Part model, mm, in its own coordinate system. Face numbers are marked on the shaded views. A direction names the side the tool comes from. Round coordinates to 2 decimals unless told otherwise and drop trailing zeros. Write each loop counter-clockwise with the first axis right and the second up, starting at its lowest first coordinate (ties: lowest second). Pieces come first, ordered by that corner, then holes. Notation, with made-up numbers: (11, 84.5) -> (48, 84.5) arc R7 ccw to (48, 96.5) -> close; hole circle Ø2 at (-21, 26.5). An arc over 180 degrees is marked (long way). Return JSON: item names as keys, results as strings. Group by question number.
(1) Saw through at C-C (y = 0.3). List the corners of the cut face in (x, z).
(2) Drill centre lines: L1, parallel to Z at x = 0, y = 0.55; L2, parallel to X at y = 0.3, z = 4; L3, parallel to X at y = 0.95, z = -4. Where is each one in solid material? Low to high. Write a range as from..to.
(3) Saw through at D-D (x = 8). List the corners of the cut face in (y, z), plus the area to 3 significant figures.
(4) Tool access for the marked faces 1, 2, 3, 4 and 5: list every direction of +Z, -Z, +X, -X, +Y, -Y with a clear straight run to the whole face (end or side of a thin tool).
(5) Mould opens along Z. For the marked faces 6, 7 and 8 say: +Z half, -Z half, draft (parallel to the pull), parting line (faces both ways), or undercut.
(6) Saw through at B-B (z = -4). List the corners of the cut face in (x, y), plus the area to 3 significant figures.
(7) Saw through at A-A (z = 4). List the corners of the cut face in (x, y).
Autodesk Inventor part; units mm, degrees
ref_plane "YZ Plane" through (0, 0, 0) normal (1, 0, 0) x (0, 1, 0)
ref_plane "XZ Plane" through (0, 0, 0) normal (0, 1, 0) x (-1, 0, 0)
ref_plane "XY Plane" through (0, 0, 0) normal (0, 0, 1) x (1, 0, 0)
sketch "Sketch1" plane through (0, 0, 0) normal (0, 1, 0) x (-1, 0, 0)
  line L0 (-1.5, -4) -> (1.5, -4)
  line L1 (1.5, -4) -> (1.5, 4)
  line L2 (1.5, 4) -> (-1.5, 4)
  line L3 (-1.5, 2) -> (-1.5, -4)
  line L4 (-1.5, -4) -> (1.5, 4) construction
  line L5 (1.5, -4) -> (-1.5, 4) construction
  circle A0 centre (0, 4) radius 1.2
  circle A1 centre (0, -4) radius 1.2
  circle A2 centre (0, -4) radius 2
  circle A3 centre (0, 4) radius 2
  line L6 (-2, 2.5) -> (-8, 2.5)
  line L7 (-8, 2.5) -> (-8, 5.5)
  line L8 (-8, 5.5) -> (0, 5.5)
  line L9 (0, 5.5) -> (0, 2.5)
  circle A4 centre (-8, 4) radius 1.2
  circle A5 centre (-8, 4) radius 2
  arc A6 (-1.5, 2) -> (-2, 2.5) centre (-2, 2) ccw
  point P0 (0, 0)
  point P1 (-1.5, -2.6771)
  point P2 (1.5, -2.6771)
  point P3 (1.5, 2.6771)
  point P4 (-1.5, 2.6771)
  point P5 (-6.6771, 2.5)
  point P6 (-1.5, 2.5)
  point P7 (-1.3229, 5.5)
  point P8 (-6.6771, 5.5)
  point P9 (-8, 5.2)
  point P10 (-8, 2.8)
  dimension "d0" = 3
  dimension "linkPitchLength" = 8
  dimension "d3" = 2.4
  dimension "d4" = 4
  dimension "linkPitchWidth" = 8
  dimension "d17" = 0.5
extrude "Extrusion1" add sketch "Sketch1" along normal blind 1 contours A1 L0 L3 A2 L1 | L0 L1 A2 L3 A1 | A2 L3 A6 L6 A5 L8 A3 L1 | A3 L8 L9 A0 L2 L1 | L1 L2 A0 L9 L8 A3 | A5 L6 L7 A4 L8 | L8 L7 A4 L6 A5
sketch "Sketch2" plane through (0, 1, 0) normal (0, 1, 0) x (1, 0, 0)
  line L0 (6.6771, -2.5) -> (2, -2.5)
  arc A0 (1.5, -2) -> (2, -2.5) centre (2, -2) ccw
  line L1 (1.5, -2) -> (1.5, 2.6771)
  arc A1 (1.5, 2.6771) -> (-1.5, 2.6771) centre (0, 4) ccw
  line L2 (-1.5, 2.6771) -> (-1.5, -2.6771)
  arc A2 (-1.5, -2.6771) -> (1.3229, -5.5) centre (0, -4) ccw
  line L3 (1.3229, -5.5) -> (6.6771, -5.5)
  arc A3 (6.6771, -5.5) -> (6.6771, -2.5) centre (8, -4) ccw
  circle A4 centre (8, -4) radius 1.2
  circle A5 centre (0, 4) radius 1.2
  circle A6 centre (0, -4) radius 1.2
  point P0 (0, 0)
extrude "Extrusion2" [suppressed]
sketch "Sketch5" plane through (0, 1, 0) normal (0, 1, 0) x (1, 0, 0)
  line L0 (6.6771, -2.5) -> (2, -2.5)
  arc A0 (1.5, -2) -> (2, -2.5) centre (2, -2) ccw
  line L1 (1.5, -2) -> (1.5, 2.6771)
  arc A1 (1.5, 2.6771) -> (-1.5, 2.6771) centre (0, 4) ccw
  line L2 (-1.5, 2.6771) -> (-1.5, -2.6771)
  arc A2 (-1.5, -2.6771) -> (1.3229, -5.5) centre (0, -4) ccw
  line L3 (1.3229, -5.5) -> (6.6771, -5.5)
  arc A3 (6.6771, -5.5) -> (6.6771, -2.5) centre (8, -4) ccw
  circle A4 centre (8, -4) radius 1.2
  circle A5 centre (0, 4) radius 1.2
  circle A6 centre (0, -4) radius 1.2
  point P0 (0, 0)
extrude "Extrusion3" [suppressed]
sketch "Sketch6" plane through (0, 1, 0) normal (0, 1, 0) x (1, 0, 0)
  line L0 (6.6771, -2.5) -> (2, -2.5)
  arc A0 (1.5, -2) -> (2, -2.5) centre (2, -2) ccw
  line L1 (1.5, -2) -> (1.5, 2.6771)
  arc A1 (1.5, 2.6771) -> (-1.5, 2.6771) centre (0, 4) ccw
  line L2 (-1.5, 2.6771) -> (-1.5, -2.6771)
  arc A2 (-1.5, -2.6771) -> (1.3229, -5.5) centre (0, -4) ccw
  line L3 (1.3229, -5.5) -> (6.6771, -5.5)
  arc A3 (6.6771, -5.5) -> (6.6771, -2.5) centre (8, -4) ccw
  circle A4 centre (8, -4) radius 1.2
  circle A5 centre (0, 4) radius 1.2
  circle A6 centre (0, -4) radius 1.2
  point P0 (0, 0)
extrude "Extrusion4" [suppressed]
properties part number "link-1-turn-8"
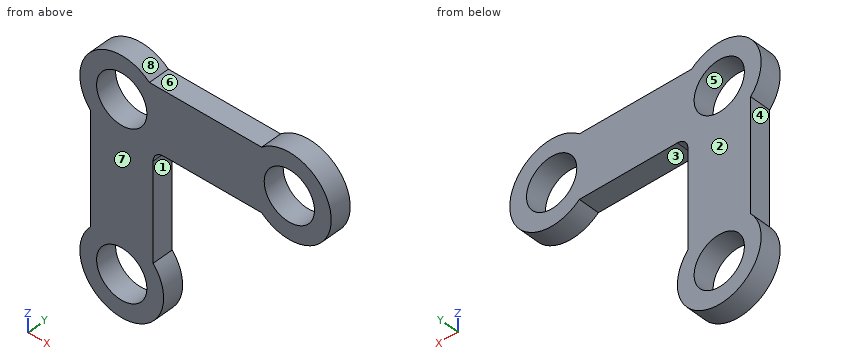
Computed values:
{
 "1": {"outline": "(-1.5, -2.68) arc R2 ccw (long way) to (1.5, -2.68) -> (1.5, 2) arc R0.5 cw to (2, 2.5) -> (6.68, 2.5) arc R2 ccw (long way) to (6.68, 5.5) -> (1.32, 5.5) arc R2 ccw to (-1.5, 2.68) -> close; hole circle Ø2.4 at (0, -4); hole circle Ø2.4 at (0, 4); hole circle Ø2.4 at (8, 4)"},
 "2": {"L1": "-6..-5.2, -2.8..2.8, 5.2..6", "L2": "-2..-1.2, 1.2..6.8, 9.2..10", "L3": "-2..-1.2, 1.2..2"},
 "3": {"outline": "(0, 2) -> (1, 2) -> (1, 2.8) -> (0, 2.8) -> close; (0, 5.2) -> (1, 5.2) -> (1, 6) -> (0, 6) -> close", "area": "1.60 mm2"},
 "4": {"face 1": "+X, +Y, -Y", "face 2": "+Z, -Z, +X, -X, +Y", "face 3": "-Z, +Y, -Y", "face 4": "-X, +Y, -Y", "face 5": "+Y, -Y"},
 "5": {"face 6": "+Z half", "face 7": "draft", "face 8": "undercut"},
 "6": {"outline": "(-2, 0) -> (-1.2, 0) -> (-1.2, 1) -> (-2, 1) -> close; (1.2, 0) -> (2, 0) -> (2, 1) -> (1.2, 1) -> close", "area": "1.60 mm2"},
 "7": {"outline": "(-2, 0) -> (-1.2, 0) -> (-1.2, 1) -> (-2, 1) -> close; (1.2, 0) -> (6.8, 0) -> (6.8, 1) -> (1.2, 1) -> close; (9.2, 0) -> (10, 0) -> (10, 1) -> (9.2, 1) -> close"}
}
